Can you work these out from the model? Positions are in its coordinate system, mm. Face numbers are marked on the shaded views. A direction names the side the tool comes from. Coordinates: 2 decimals unless noted, no trailing zeros. Order: outer loops, then holes, each group sorted by start corner. A loop starts at its lowest first (then second) coordinate and runs counter-clockwise, first axis right, second up. Notation, with made-up numbers: (32, 6.25) -> (56, 6.25) arc R17 ccw to (56, 11.25) -> close; hole circle Ø6 at (-15.5, 19.5). An arc over 180 degrees is marked (long way). Use a Markdown table: item, result. Add a question column.
1. Suppose I cut it at A-A, the plane x = 0. List the corners of the cut face in (y, z) for me.
2. If I drill on line 1 along Y through (x, z) = (-0.5, 19); line 2 along Z through (x, y) = (-2.5, -26); line 3 along X through (y, z) = (2.5, 85), over which ranges is the centre line in solid material (lowest first)? Write a range as from..to.
3. For pin 1 Ø1.5 at (y, z) = (-9, 27) entering from -X; pin 2 Ø12 at (x, z) = (10, 50) entering from -Y; pin 3 Ø6 at (x, z) = (19.5, 16) entering from -Y, each with a flat end and sliding along its axis, tell me the tip position at first contact or that it passes through.
4. For the marked faces 1 and 2, which set-ups out of +Z, -Z, +X, -X, +Y, -Y let a thin tool reach every point of the face, with its end or its side?
5. Suppose I cut it at C-C, the plane z = 91.5. List the corners of the cut face in (x, y) for me.
```python
from build123d import *

# Parameters (mm, degrees)
SKETCH2_R           = 20
BOSS_EXTRUDE1_DEPTH = 100
SKETCH3_R           = 40
BOSS_EXTRUDE2_DEPTH = 5
CHAMFER1_SIZE       = 2


with BuildPart() as part:
    # Sketch2 → Boss-Extrude1 (new body)
    with BuildSketch(Plane.XY):
        Circle(SKETCH2_R)
    extrude(amount=BOSS_EXTRUDE1_DEPTH)

    # Sketch3 → Boss-Extrude2 (add)
    with BuildSketch(Plane(origin=(0, 0, 0), x_dir=(-1, 0, 0), z_dir=(0, 0, -1))):
        Circle(SKETCH3_R)
    extrude(amount=BOSS_EXTRUDE2_DEPTH)

    # Chamfer1
    chamfer1_edges = [part.edges().sort_by_distance(p)[0] for p in [
        (40, 0, -5),
    ]]
    chamfer(chamfer1_edges, length=CHAMFER1_SIZE)


solid = part.part
```
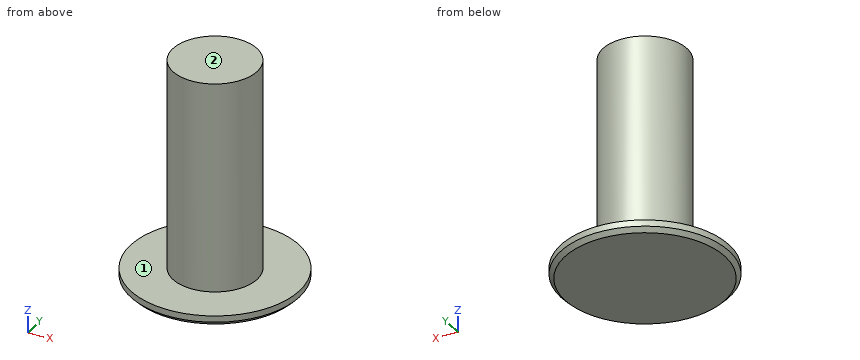
Worked out:
| question | item | result |
|---|---|---|
| 1 | outline | (-40, -3) -> (-38, -5) -> (38, -5) -> (40, -3) -> (40, 0) -> (20, 0) -> (20, 100) -> (-20, 100) -> (-20, 0) -> (-40, 0) -> close |
| 2 | line 1 | y = -19.99..19.99 |
| 2 | line 2 | z = -5..0 |
| 2 | line 3 | x = -19.84..19.84 |
| 3 | pin 1 | stops at x = -18.22 |
| 3 | pin 2 | stops at y = -19.6 |
| 3 | pin 3 | stops at y = -11.3 |
| 4 | face 1 | +Z |
| 4 | face 2 | +Z, +X, -X, +Y, -Y |
| 5 | outline | circle Ø40 at (0, 0) |
